Autodesk Inventor part; units mm, degrees
ref_plane "YZ Plane" through (0, 0, 0) normal (1, 0, 0) x (0, 1, 0)
ref_plane "XZ Plane" through (0, 0, 0) normal (0, 1, 0) x (-1, 0, 0)
ref_plane "XY Plane" through (0, 0, 0) normal (0, 0, 1) x (1, 0, 0)
sketch "Sketch1" plane through (0, 0, 0) normal (0, 0, 1) x (1, 0, 0)
  circle A0 centre (-17.5, -17.5) radius 1.5
  circle A1 centre (17.5, -17.5) radius 1.5
  circle A2 centre (17.5, 17.5) radius 1.5
  circle A3 centre (-17.5, 17.5) radius 1.5
  line L0 (-22.5, 22.5) -> (22.5, 22.5)
  line L1 (22.5, 22.5) -> (22.5, -22.5)
  line L2 (22.5, -22.5) -> (-22.5, -22.5)
  line L3 (-22.5, -22.5) -> (-22.5, 22.5)
  point P0 (0, 0)
  dimension "d4" = 3
  dimension "d5" = 3
  dimension "d6" = 3
  dimension "d7" = 3
  dimension "d8" = 35
  dimension "d9" = 35
  dimension "d10" = 35
  dimension "d13" = 45
  dimension "d14" = 45
  dimension "d15" = 22.5
  dimension "d16" = 22.5
  dimension "d17" = 5
  dimension "d18" = 5
sketch "Sketch2" plane through (0, 0, 0) normal (0, 0, 1) x (1, 0, 0)
  line L0 (-30, 30) -> (30, 30)
  line L1 (30, 30) -> (30, -30)
  line L2 (30, -30) -> (-30, -30)
  line L3 (-30, -30) -> (-30, 30)
  point P0 (0, 0)
  dimension "d20" = 60
  dimension "d21" = 60
  dimension "d22" = 30
  dimension "d23" = 30
extrude "Extrusion1" add sketch "Sketch2" along normal blind 18.5
extrude "Extrusion2" cut sketch "Sketch1" along normal blind 18
sketch "Sketch3" plane through (-17.5, 17.5, 0) normal (0, 0, -1) x (-1, 0, 0)
  circle A0 centre (0, 0) radius 1.5
  circle A1 centre (0, -35) radius 1.5
  circle A2 centre (-35, 0) radius 1.5
  circle A3 centre (-35, -35) radius 1.5
  point P0 (-17.5, -17.5)
extrude "Extrusion3" cut sketch "Sketch3" against normal blind 19
properties part number "soporte_iman"
Here's how the part is built. I have some questions about the finished solid (model axes, mm). A direction names the side the tool comes from. Give positions to 0.01 mm unless a question says otherwise; leave off trailing zeros. Order: outer loops, then holes, each group sorted by start corner. A loop starts at its lowest first (then second) coordinate and runs counter-clockwise, first axis right, second up. Notation, with made-up numbers: (-3, 21.25) -> (43, 21.25) arc R15 cw to (43, 31.25) -> close; hole circle Ø5 at (6.5, 23). An arc over 180 degrees is marked (long way). Use a Markdown table: item, result. Add a question column.
Item 1: Imagine slicing it at B-B on x = -17.5. Please give me the cut outline in (y, z).
Item 2: Will this pin go through, and if not, where does the flat tip stop? pin 1 (22.5 mm diameter, centred on x = 9, y = -9, fed in from -Z).
Item 3: For faces 1 (the face through (-16, -17.43, 18.25)), 2 (the face through (0, 0, 18)), which set-ups out of +Z, -Z, +X, -X, +Y, -Y let a thin tool reach every point of the face, with its end or its side?
Item 4: I need wall thicknesses on line 1 (Y direction, x = -17.5, z = 18.2); line 2 (X direction, y = 16, z = 8.25). Which ranges of each line are inside material? Lowest first, please.
Item 5: If we mould it in two halves opening along Y, with no side actions, what happens to faces 3 (the face through (-22.5, 0, 9)), 4 (the face through (0, 30, 9)), 5 (the face through (-27, 0, 0))? For each: pulls with the +Y half, pulls with the -Y half, needs draft (parallel to the pull), parting line crosses it, or undercut.
Item 6: Imagine slicing it at A-A on z = 3.5. Please give me the cut outline in (x, y).
Item 7: Imagine slicing it at D-D on x = -5. Please give me the cut outline in (y, z).
Data:
| question | item | result |
|---|---|---|
| 1 | outline | (-30, 0) -> (-22.5, 0) -> (-22.5, 18) -> (-19, 18) -> (-19, 18.5) -> (-30, 18.5) -> close; (-16, 18) -> (16, 18) -> (16, 18.5) -> (-16, 18.5) -> close; (19, 18) -> (22.5, 18) -> (22.5, 0) -> (30, 0) -> (30, 18.5) -> (19, 18.5) -> close |
| 2 | pin 1 | stops at z = 18 |
| 3 | face 1 | +Z, -Z |
| 3 | face 2 | -Z |
| 4 | line 1 | y = -30 to -19, -16 to 16, 19 to 30 |
| 4 | line 2 | x = -30 to -22.5, 22.5 to 30 |
| 5 | face 3 | undercut |
| 5 | face 4 | pulls with the +Y half |
| 5 | face 5 | needs draft |
| 6 | outline | (-30, -30) -> (30, -30) -> (30, 30) -> (-30, 30) -> close; hole (-22.5, -22.5) -> (22.5, -22.5) -> (22.5, 22.5) -> (-22.5, 22.5) -> close |
| 7 | outline | (-30, 0) -> (-22.5, 0) -> (-22.5, 18) -> (22.5, 18) -> (22.5, 0) -> (30, 0) -> (30, 18.5) -> (-30, 18.5) -> close |
